Can you work these out from the model? Positions are in its coordinate system, mm. Face numbers are marked on the shaded views. A direction names the side the tool comes from. Give positions to 0.01 mm unless a question says otherwise; leave off trailing zeros. Loops run counter-clockwise (first coordinate to the right, second up) from the corner with the lowest first, then second, coordinate; pieces in that order, holes last. Notation, with made-up numbers: M -30,3 L -7,3 A28 cw -7,36 Z; hole C 15,78.25 d8. An arc over 180 degrees is marked long. Answer as a JSON object with one key per item and string values.
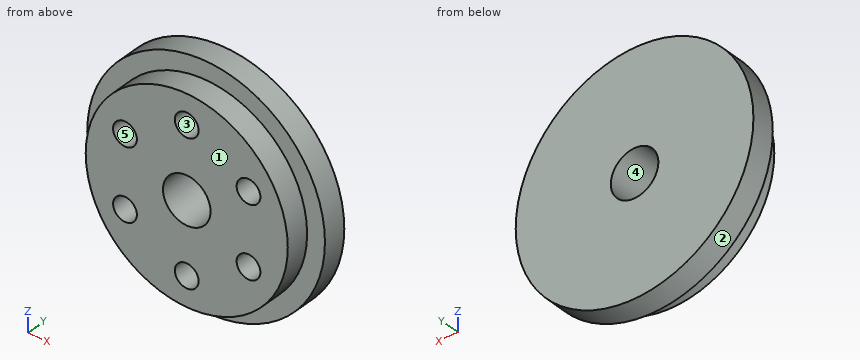
```python
from build123d import *

# Parameters (mm, degrees)
F0_R     = 8.5
F0_R_2   = 1
F1_DEPTH = 2
F2_R     = 10
F3_DEPTH = 2
F4_R     = 2
F5_DEPTH = 4.001


with BuildPart() as f1:
    # F0 (on Front) → F1 (new body)
    with BuildSketch(Plane.XZ):
        Circle(F0_R)
        with Locations((-5.196152, -3)):
            Circle(F0_R_2, mode=Mode.SUBTRACT)
        with Locations((0, -6)):
            Circle(F0_R_2, mode=Mode.SUBTRACT)
        with Locations((5.196152, -3)):
            Circle(F0_R_2, mode=Mode.SUBTRACT)
        with Locations((-5.196152, 3)):
            Circle(F0_R_2, mode=Mode.SUBTRACT)
        with Locations((5.196152, 3)):
            Circle(F0_R_2, mode=Mode.SUBTRACT)
        with Locations((0, 6)):
            Circle(F0_R_2, mode=Mode.SUBTRACT)
    extrude(amount=F1_DEPTH)

    # F2 (on face) → F3 (join)
    with BuildSketch(Plane(origin=(0, 0, 0), x_dir=(-1, 0, 0), z_dir=(0, 1, 0))):
        Circle(F2_R)
    extrude(amount=F3_DEPTH)

    # F4 (on face) → F5 (cut, through all)
    with BuildSketch(Plane.XZ.offset(2)):
        Circle(F4_R)
    extrude(amount=-F5_DEPTH, mode=Mode.SUBTRACT)


solid = f1.part
```
1) Please list where these lines run through material, in increasing order: line 1 along Z through (x, y) = (5, -0.1); line 2 along X through (y, z) = (-1.65, 2.75); line 3 along Z through (x, y) = (0, -1.55). Write a range as from..to.
Answer list:
{"line 1": "-6.87..-3.98, -2.02..2.02, 3.98..6.87", "line 2": "-8.04..-6.16, -4.23..4.23, 6.16..8.04", "line 3": "-8.5..-7, -5..-2, 2..5, 7..8.5"}
2) Suppose I cut it at A-A, the plane z = 0. Write out the boundary of the cut face in (x, y), and give its area (3 significant figures).
Answer list:
{"outline": "M -10,0 L -8.5,0 L -8.5,-2 L -2,-2 L -2,2 L -10,2 Z; M 2,-2 L 8.5,-2 L 8.5,0 L 10,0 L 10,2 L 2,2 Z", "area": "58.0 mm^2"}
3) If we mould it in two halves opening along X, with no side actions, what happens to the marked faces 1, 2 and 3? For each: +X half, -X half, draft (parallel to the pull), parting line (faces both ways), or undercut.
Answer list:
{"face 1": "draft", "face 2": "parting line", "face 3": "undercut"}
4) For the marked faces 4 and 5, which set-ups out of +Z, -Z, +X, -X, +Y, -Y let a thin tool reach every point of the face, with its end or its side?
Answer list:
{"face 4": "+Y, -Y", "face 5": "-Y"}
5) Will these pins go through, and if not, where does the flat tip stop? pin 1 Ø1 at (x, z) = (0, -6) entering from -Y; pin 2 Ø1 at (y, z) = (1, 3) entering from +X; pin 3 Ø2 at (y, z) = (0, -7) entering from -X.
Answer list:
{"pin 1": "y = 0", "pin 2": "x = 9.68", "pin 3": "x = -8"}
6) Suppose I cut it at B-B, the plane x = 0. Write out the boundary of the cut face in (y, z).
Answer list:
{"outline": "M -2,-8.5 L 0,-8.5 L 0,-10 L 2,-10 L 2,-2 L -2,-2 L -2,-5 L 0,-5 L 0,-7 L -2,-7 Z; M -2,2 L 2,2 L 2,10 L 0,10 L 0,8.5 L -2,8.5 L -2,7 L 0,7 L 0,5 L -2,5 Z"}
7) Suppose I cut it at C-C, the plane y = -0.65. Write out the boundary of the cut face in (x, z), and give its area (3 significant figures).
Answer list:
{"outline": "C 0,0 d17; hole C -5.2,-3 d2; hole C -5.2,3 d2; hole C 0,0 d4; hole C 0,-6 d2; hole C 0,6 d2; hole C 5.2,-3 d2; hole C 5.2,3 d2", "area": "196 mm^2"}
8) Suppose I cut it at D-D, the plane z = 6. Write out the boundary of the cut face in (x, y), and give its area (3 significant figures).
Answer list:
{"outline": "M -8,0 L -6.02,0 L -6.02,-2 L -1,-2 L -1,0 L 1,0 L 1,-2 L 6.02,-2 L 6.02,0 L 8,0 L 8,2 L -8,2 Z", "area": "52.1 mm^2"}
